Verification items for this drawing (mm, ordinates from the low corner). A direction names the side the tool comes from. Round coordinates to 2 decimals unless told otherwise and drop trailing zeros. Order: outer loops, then holes, each group sorted by start corner. A loop starts at its lowest first (then second) coordinate and runs counter-clockwise, first axis right, second up. Notation, with made-up numbers: (47, -35.75) -> (56, -35.75) arc R18 cw to (56, -10.75) -> close; hole circle Ø6 at (31, -38). An arc over 180 degrees is marked (long way). Return JSON: item names as keys, results as strings. Group by question number.
Item 1: Depth check by flat-ended pin: pin 1 Ø2 at (x, z) = (37, 12.5) entering from -Y; pin 2 Ø5 at (y, z) = (31.5, 25) entering from -X; pin 3 Ø12 at (x, y) = (18.5, 37) entering from +Z; pin 4 Ø8 at (y, z) = (30, 13) entering from +X. Enter the tip coordinate at first touch or a pass-through.
Item 2: Sectioned sample at D-D on z = 7. Record the cut outline in (x, y).
Item 3: Scan lines: probe 1 along Y at (x, z) = (74, 12); probe 2 along X at (y, z) = (30.5, 10.5); probe 3 along Z at (x, y) = (45, 27). Record each from-to range of solid material in increasing order. Write a range as from..to.
Item 4: Sectioned sample at A-A on z = 39. Record the cut outline in (x, y).
Item 5: Access from +Z, -Z, +X, -X, +Y, -Y to the whole of each face (thin tool, end or side, straight path). Record for the marked faces 1, 2 and 3.
Item 6: Sectioned sample at C-C on x = 8.5. Record the cut outline in (y, z), plus the area to 3 significant figures.
Item 7: Sectioned sample at B-B on y = 41.5. Record the cut outline in (x, z).
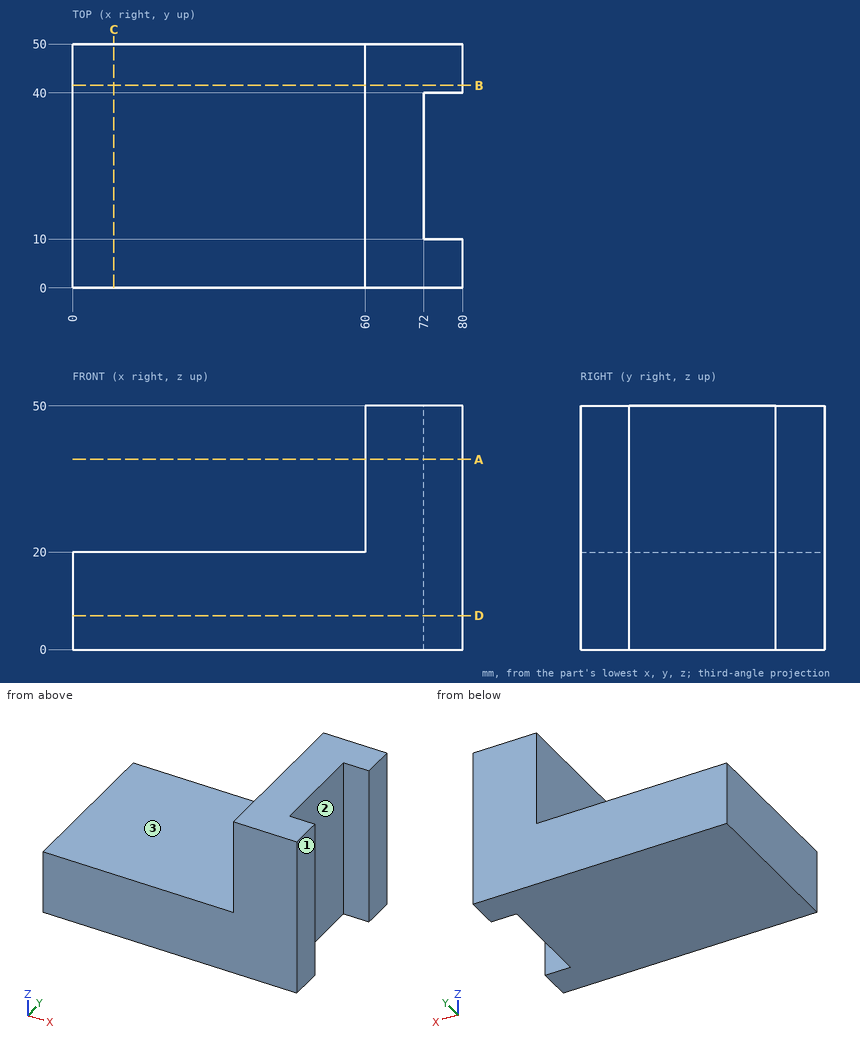
Recorded:
{
 "1": {"pin 1": "y = 0", "pin 2": "x = 60", "pin 3": "z = 20", "pin 4": "x = 72"},
 "2": {"outline": "(0, 0) -> (80, 0) -> (80, 10) -> (72, 10) -> (72, 40) -> (80, 40) -> (80, 50) -> (0, 50) -> close"},
 "3": {"probe 1": "0..10, 40..50", "probe 2": "0..72", "probe 3": "0..20"},
 "4": {"outline": "(60, 0) -> (80, 0) -> (80, 10) -> (72, 10) -> (72, 40) -> (80, 40) -> (80, 50) -> (60, 50) -> close"},
 "5": {"face 1": "+Z, -Z, +X, +Y, -Y", "face 2": "+Z, -Z, +X", "face 3": "+Z, -X, +Y, -Y"},
 "6": {"outline": "(0, 0) -> (50, 0) -> (50, 20) -> (0, 20) -> close", "area": "1,000 mm²"},
 "7": {"outline": "(0, 0) -> (80, 0) -> (80, 50) -> (60, 50) -> (60, 20) -> (0, 20) -> close"}
}
